The listing builds one solid part. Answer for the finished solid, in the listing's coordinates (mm). Face numbers are marked on the shaded views. A direction names the side the tool comes from. Round coordinates to 2 decimals unless told otherwise and drop trailing zeros. Write each loop counter-clockwise with the first axis right and the second up, starting at its lowest first coordinate (ties: lowest second). Pieces come first, ordered by that corner, then holes. Notation, with made-up numbers: M 6.25,87.25 L 10.25,87.25 A19 ccw 10.25,102.25 Z; hole C 40.5,-15 d8. An arc over 180 degrees is marked long. Write each question's results on one line, items separated by ' | '.
from build123d import *

# Parameters (mm, degrees)
ESQUISSE2_W                   = 170
ESQUISSE2_H                   = 150
BOSS_EXTRU_1_DEPTH            = 35
ESQUISSE3_R                   = 42.75
ENL_V_MAT_EXTRU_2_DEPTH       = 40
ESQUISSE5_R                   = 6
ENL_V_MAT_EXTRU_3_DEPTH       = 40
ESQUISSE6_R                   = 9.5
ENL_V_MAT_EXTRU_4_DEPTH       = 13
ESQUISSE7_R                   = 5.25
ENL_V_MAT_EXTRU_5_DEPTH       = 40
ESQUISSE8_R                   = 8.5
ENL_V_MAT_EXTRU_6_DEPTH       = 11
ESQUISSE9_R                   = 4.25
ENL_V_MAT_EXTRU_7_DEPTH       = 25
ENL_V_MAT_EXTRU_8_DEPTH       = 1
ENL_V_MAT_EXTRU_8_DEPTH_BACK  = 36
ENL_V_MAT_EXTRU_12_DEPTH      = 1
ENL_V_MAT_EXTRU_12_DEPTH_BACK = 36
ENL_V_MAT_EXTRU_13_DEPTH      = 1
ENL_V_MAT_EXTRU_13_DEPTH_BACK = 36
ENL_V_MAT_EXTRU_14_DEPTH      = 1
ENL_V_MAT_EXTRU_14_DEPTH_BACK = 36
CONG_1_R                      = 10
CONG_2_R                      = 10
CONG_3_R                      = 10
CONG_4_R                      = 10
CONG_5_R                      = 2
ENL_V_MAT_EXTRU_17_DEPTH      = 10


with BuildPart() as part:
    # Esquisse2 → Boss.-Extru.1 (new body)
    with BuildSketch(Plane.XY):
        with Locations((-85, 75)):
            Rectangle(ESQUISSE2_W, ESQUISSE2_H)
    extrude(amount=BOSS_EXTRU_1_DEPTH)

    # Esquisse3 → Enlèv. mat.-Extru.2 (cut)
    with BuildSketch(Plane.XY.offset(35)):
        with Locations((-85, 75)):
            Circle(ESQUISSE3_R)
    extrude(amount=-ENL_V_MAT_EXTRU_2_DEPTH, mode=Mode.SUBTRACT)

    # Esquisse5 → Enlèv. mat.-Extru.3 (cut)
    with BuildSketch(Plane.XY.offset(35)):
        with Locations((-38.5, 101.5)):
            Circle(ESQUISSE5_R)
        with Locations((-38.5, 48.5)):
            Circle(ESQUISSE5_R)
        with Locations((-131.5, 48.5)):
            Circle(ESQUISSE5_R)
        with Locations((-131.5, 101.5)):
            Circle(ESQUISSE5_R)
    extrude(amount=-ENL_V_MAT_EXTRU_3_DEPTH, mode=Mode.SUBTRACT)

    # Esquisse6 → Enlèv. mat.-Extru.4 (cut)
    with BuildSketch(Plane.XY.offset(35)):
        with Locations((-38.5, 101.5)):
            Circle(ESQUISSE6_R)
        with Locations((-38.5, 48.5)):
            Circle(ESQUISSE6_R)
        with Locations((-131.5, 48.5)):
            Circle(ESQUISSE6_R)
        with Locations((-131.5, 101.5)):
            Circle(ESQUISSE6_R)
    extrude(amount=-ENL_V_MAT_EXTRU_4_DEPTH, mode=Mode.SUBTRACT)

    # Esquisse7 → Enlèv. mat.-Extru.5 (cut)
    with BuildSketch(Plane.XY.offset(35)):
        with Locations((-11, 139)):
            Circle(ESQUISSE7_R)
        with Locations((-11, 11)):
            Circle(ESQUISSE7_R)
        with Locations((-159, 11)):
            Circle(ESQUISSE7_R)
        with Locations((-159, 139)):
            Circle(ESQUISSE7_R)
    extrude(amount=-ENL_V_MAT_EXTRU_5_DEPTH, mode=Mode.SUBTRACT)

    # Esquisse8 → Enlèv. mat.-Extru.6 (cut)
    with BuildSketch(Plane.XY.offset(35)):
        with Locations((-11, 139)):
            Circle(ESQUISSE8_R)
        with Locations((-11, 11)):
            Circle(ESQUISSE8_R)
        with Locations((-159, 11)):
            Circle(ESQUISSE8_R)
        with Locations((-159, 139)):
            Circle(ESQUISSE8_R)
    extrude(amount=-ENL_V_MAT_EXTRU_6_DEPTH, mode=Mode.SUBTRACT)

    # Esquisse9 → Enlèv. mat.-Extru.7 (cut)
    with BuildSketch(Plane(origin=(0, 150, 0), x_dir=(1, 0, 0), z_dir=(0, 1, 0))):
        with Locations(Location((-25, -23, 0), (0, 0, 270))):  # turned: the seam where the file's is
            Circle(ESQUISSE9_R)
        with Locations(Location((-145, -23, 0), (0, 0, 270))):  # turned: the seam where the file's is
            Circle(ESQUISSE9_R)
    extrude(amount=-ENL_V_MAT_EXTRU_7_DEPTH, mode=Mode.SUBTRACT)

    # Esquisse19 → Enlèv. mat.-Extru.8 (cut, two sides)
    with BuildSketch(Plane.XY.offset(35)) as enl_v_mat_extru_8_sk:
        with BuildLine():
            Line((348.687033491, 365.032270311), (0, 120))
            ThreePointArc((0, 120), (-23.377223398, 75), (0, 30))
            Line((0, 30), (348.687033491, -215.032270311))
            Line((348.687033491, -215.032270311), (1201.033115359, -215.032270311))
            Line((1201.033115359, -215.032270311), (1201.033115359, 365.032270311))
            Line((1201.033115359, 365.032270311), (348.687033491, 365.032270311))
        make_face()
    extrude(amount=ENL_V_MAT_EXTRU_8_DEPTH, mode=Mode.SUBTRACT)
    extrude(enl_v_mat_extru_8_sk.sketch, amount=-ENL_V_MAT_EXTRU_8_DEPTH_BACK, mode=Mode.SUBTRACT)

    # Esquisse22 → Enlèv. mat.-Extru.12 (cut, two sides)
    with BuildSketch(Plane.XY.offset(35)) as enl_v_mat_extru_12_sk:
        with BuildLine():
            Line((-498.703585548, -196.956534006), (-135, 0))
            ThreePointArc((-135, 0), (-85, 12.669073437), (-35, 0))
            Line((-35, 0), (328.703585548, -196.956534006))
            Line((328.703585548, -196.956534006), (328.703585548, -1024.17397683))
            Line((328.703585548, -1024.17397683), (-498.703585548, -1024.17397683))
            Line((-498.703585548, -1024.17397683), (-498.703585548, -196.956534006))
        make_face()
    extrude(amount=ENL_V_MAT_EXTRU_12_DEPTH, mode=Mode.SUBTRACT)
    extrude(enl_v_mat_extru_12_sk.sketch, amount=-ENL_V_MAT_EXTRU_12_DEPTH_BACK, mode=Mode.SUBTRACT)

    # Esquisse27 → Enlèv. mat.-Extru.13 (cut, two sides)
    with BuildSketch(Plane.XY.offset(35)) as enl_v_mat_extru_13_sk:
        with BuildLine():
            Line((-518.687033491, 365.032270311), (-170, 120))
            ThreePointArc((-170, 120), (-146.622776602, 75), (-170, 30))
            Line((-170, 30), (-518.687033491, -215.032270311))
            Line((-518.687033491, -215.032270311), (-1371.033115359, -215.032270311))
            Line((-1371.033115359, -215.032270311), (-1371.033115359, 365.032270311))
            Line((-1371.033115359, 365.032270311), (-518.687033491, 365.032270311))
        make_face()
    extrude(amount=ENL_V_MAT_EXTRU_13_DEPTH, mode=Mode.SUBTRACT)
    extrude(enl_v_mat_extru_13_sk.sketch, amount=-ENL_V_MAT_EXTRU_13_DEPTH_BACK, mode=Mode.SUBTRACT)

    # Esquisse28 → Enlèv. mat.-Extru.14 (cut, two sides)
    with BuildSketch(Plane.XY.offset(35)) as enl_v_mat_extru_14_sk:
        with BuildLine():
            Line((-498.703585548, 346.956534006), (-135, 150))
            ThreePointArc((-135, 150), (-85, 137.330926563), (-35, 150))
            Line((-35, 150), (328.703585548, 346.956534006))
            Line((328.703585548, 346.956534006), (328.703585548, 1174.17397683))
            Line((328.703585548, 1174.17397683), (-498.703585548, 1174.17397683))
            Line((-498.703585548, 1174.17397683), (-498.703585548, 346.956534006))
        make_face()
    extrude(amount=ENL_V_MAT_EXTRU_14_DEPTH, mode=Mode.SUBTRACT)
    extrude(enl_v_mat_extru_14_sk.sketch, amount=-ENL_V_MAT_EXTRU_14_DEPTH_BACK, mode=Mode.SUBTRACT)

    # Congé1
    cong_1_edges = [part.edges().sort_by_distance(p)[0] for p in [
        (0, 150, 17.5),
    ]]
    fillet(cong_1_edges, radius=CONG_1_R)

    # Congé2
    cong_2_edges = [part.edges().sort_by_distance(p)[0] for p in [
        (-170, 150, 17.5),
    ]]
    fillet(cong_2_edges, radius=CONG_2_R)

    # Congé3
    cong_3_edges = [part.edges().sort_by_distance(p)[0] for p in [
        (-170, 0, 17.5),
    ]]
    fillet(cong_3_edges, radius=CONG_3_R)

    # Congé4
    cong_4_edges = [part.edges().sort_by_distance(p)[0] for p in [
        (0, 0, 17.5),
    ]]
    fillet(cong_4_edges, radius=CONG_4_R)

    # Congé5
    cong_5_edges = [part.edges().sort_by_distance(p)[0] for p in [
        (-127.75, 75, 0),
    ]]
    fillet(cong_5_edges, radius=CONG_5_R)

    # Esquisse40 → Enlèv. mat.-Extru.17 (cut)
    with BuildSketch(Plane.XY.offset(35)):
        with BuildLine():
            Line((-135, 150), (-135, 137))
            Line((-135, 137), (-35, 137))
            Line((-35, 137), (-35, 150))
            ThreePointArc((-35, 150), (-85, 137.330926563), (-135, 150))
        make_face()
    extrude(amount=-ENL_V_MAT_EXTRU_17_DEPTH, mode=Mode.SUBTRACT)


solid = part.part
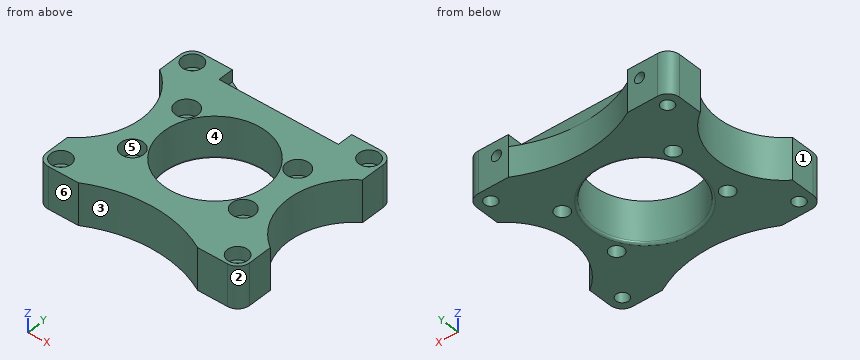
1) A tool of negligible diameter and unlimited length cuts with its end or side. For the marked faces 5 and 6, from which of +Z, -Z, +X, -X, +Y, -Y can it reach the whole face along a straight path? Write none if from no direction.
Return value:
face 5: +Z | face 6: +Z, -Z, +X, -X, -Y
2) Section A-A (x = -85) is taken. Determine the outline of the cut face in (y, z), then the cut area to 3 significant figures.
Return value:
outline: M 12.67,0 L 30.25,0 A2 ccw 32.25,2 L 32.25,35 L 12.67,35 Z; M 117.75,2 A2 ccw 119.75,0 L 137.33,0 L 137.33,25 L 137,25 L 137,35 L 117.75,35 Z | area: 1,370 mm²
3) Find the intervals of material crossed by line 1 (X direction, y = 137, z = 23); line 2 (Y direction, x = -36, z = 18); line 3 (Y direction, x = -38, z = 30), in increasing order.
Return value:
line 1: -170 to -163.85, -154.15 to -149.25, -140.75 to -29.25, -20.75 to -15.85, -6.15 to 0 | line 2: 0.53 to 43.05, 53.95 to 96.05, 106.95 to 149.47 | line 3: 1.56 to 39.01, 57.99 to 92.01, 110.99 to 137
4) Each of these flat-tipped pins is pushed along its axis until it touches: pin 1 (7 mm diameter, centred on x = -38.5, y = 48.5, fed in from +Z); pin 2 (1.5 mm diameter, centred on x = -87, z = 4, fed in from +Y); pin 3 (15 mm diameter, centred on x = -131.5, y = 48.5, fed in from +Z); pin 4 (8 mm diameter, centred on x = -77.5, y = 29.5, fed in from -Z). Where does it stop, or does it pass through?
Return value:
pin 1: through | pin 2: y = 137.37 | pin 3: z = 22 | pin 4: z = 0
5) Section B-B (z = 29.5) is taken. State how many separate pieces and enclosed holes the cut face has, then the cut area to 3 significant figures.
Return value:
separate pieces: 1 | enclosed holes: 9 | area: 12,500 mm²
6) The mould has two halves that part along X. Classify the marked faces 1, 2, 3 and 4: +X half, -X half, draft (parallel to the pull), parting line (faces both ways), or undercut.
Return value:
face 1: -X half | face 2: +X half | face 3: undercut | face 4: undercut
